```python
from build123d import *

# Parameters (mm, degrees)
F1_DEPTH = 100
F2_W     = 176
F2_H     = 188
F3_DEPTH = 200.001


with BuildPart() as f1:
    # F0 (on Front) → F1 (new body, symmetric)
    with BuildSketch(Plane.XZ):
        Polygon((-88, 200), (-94, 200), (-94, 6), (94, 6), (94, 200), (88, 200), (88, 12), (-88, 12), align=None)
        Polygon((-100, 200), (-100, 0), (100, 0), (100, 200), (94, 200), (94, 6), (-94, 6), (-94, 200), align=None)
    extrude(amount=F1_DEPTH, both=True)

    # F2 (on face) → F3 (cut, through all)
    with BuildSketch(Plane.YZ.offset(100)):
        with Locations((0, 94)):
            Rectangle(F2_W, F2_H)
    extrude(amount=-F3_DEPTH, mode=Mode.SUBTRACT)


solid = f1.part
```
The model under review builds one solid part; all positions refer to its coordinate system, in mm. A direction names the side the tool comes from. Round coordinates to 2 decimals unless told otherwise and drop trailing zeros. Write each loop counter-clockwise with the first axis right and the second up, starting at its lowest first coordinate (ties: lowest second). Pieces come first, ordered by that corner, then holes. Notation, with made-up numbers: (20.25, 66) - (34.25, 66) arc R18 ccw to (34.25, 95) - close; hole circle Ø9 at (-5, 26). An arc over 180 degrees is marked (long way). Use one line per item in the form item = value.
Q1. For line 1 (Y direction, x = -8, z = 11); line 2 (Z direction, x = 70, y = -90), list the stretches that pass through material, from the lowest coordinate up. Write a range as [from, to].
Answer key:
line_1 = [-100, -88], [88, 100]
line_2 = [0, 12]
Q2. Tool access review of faces 5 (the flat face through (-0.5, 100, 11.6)), 6 (the flat face through (-7, -88, 10)), 7 (the flat face through (1, 94, 12)): name each direction out of +Z, -Z, +X, -X, +Y, -Y from which nothing blocks a thin tool from reaching the whole face with its end or side.
Answer key:
face_5 = +Z, -Z, +X, -X, +Y
face_6 = -Z, +X, -X
face_7 = +Z, +Y, -Y
Q3. Insertion check: pin 1 Ø13 at (x, y) = (-21.5, -96) entering from +Z; pin 2 Ø13 at (x, y) = (97, 13.5) entering from -Z. Each pin has a flat end and moves straight along its axis. Give the tip position at first contact, or say it passes through.
Answer key:
pin_1 = 12
pin_2 = 188
Q4. Consider section A-A (x = 67). State the section outline as (y, z) points, and give its area (3 significant figures).
Answer key:
outline = (-100, 0) - (-88, 0) - (-88, 12) - (-100, 12) - close; (88, 0) - (100, 0) - (100, 12) - (88, 12) - close
area = 288 mm2
Q5. Consider section B-B (z = 148). State the section outline as (x, y) points, and give its area (3 significant figures).
Answer key:
outline = (-100, -100) - (-88, -100) - (-88, -88) - (-100, -88) - close; (-100, 88) - (-88, 88) - (-88, 100) - (-100, 100) - close; (88, -100) - (100, -100) - (100, -88) - (88, -88) - close; (88, 88) - (100, 88) - (100, 100) - (88, 100) - close
area = 576 mm2
Q6. Consider section C-C (y = -66). State the section outline as (x, z) points.
Answer key:
outline = (-100, 188) - (-88, 188) - (-88, 200) - (-100, 200) - close; (88, 188) - (100, 188) - (100, 200) - (88, 200) - close
Q7. Draft analysis for pull direction X (two halves, no side actions). For faces 1 (the flat face through (-7, 88, 10)), 2 (the flat face through (88, 7, 190)), 3 (the flat face through (1, -94, 12)), 4 (the flat face through (-100, 7, 189)), state which applies: +X half, -X half, draft (parallel to the pull), parting line (faces both ways), or undercut.
Answer key:
face_1 = draft
face_2 = undercut
face_3 = undercut
face_4 = -X half
